```python
from build123d import *

# Parameters (mm, degrees)
BOSS_EXTRUDE2_DEPTH      = 10
SKETCH2_R                = 3
CUT_EXTRUDE1_DEPTH       = 5
CUT_EXTRUDE2_REACH       = 40.514
SKETCH3_R                = 1.5
SKETCH4_W                = 28.86751346
SKETCH4_H                = 120
SKETCH4_R                = 1.5
BOSS_EXTRUDE4_DEPTH      = 10
SKETCH5_R                = 3
CUT_EXTRUDE3_DEPTH       = 5
SKETCH6_W                = 4
SKETCH6_H                = 2
SKETCH6_W_2              = 2
SKETCH6_H_2              = 4
CUT_EXTRUDE4_DEPTH       = 4
SKETCH7_R                = 14.43375673
BOSS_EXTRUDE5_DEPTH      = 60
SKETCH8_R                = 9.43375673
CUT_EXTRUDE6_DEPTH       = 120
BOSS_EXTRUDE6_REACH      = 167.526
BOSS_EXTRUDE6_END_RADIUS = 14.43375673
SKETCH11_W               = 28.86751346
SKETCH11_H               = 10
CUT_EXTRUDE7_REACH       = 167.526
SKETCH13_W               = 18.86751346
SKETCH13_H               = 50
FILLET3_R                = 2
FILLET4_R                = 2


with BuildPart() as part:
    # Sketch1 → Boss-Extrude2 (new body)
    with BuildSketch(Plane.XY):
        Polygon((14.43375673, 25), (-14.43375673, 25), (-28.867513459, 0), (-14.43375673, -25), (14.43375673, -25), (28.867513459, 0), align=None)
    extrude(amount=BOSS_EXTRUDE2_DEPTH)

    # Sketch2 → Cut-Extrude1 (cut)
    with BuildSketch(Plane.XY.offset(10)):
        with Locations((-5.480077554, 5.480077554)):
            Circle(SKETCH2_R)
        with Locations((6.717514421, 6.717514421)):
            Circle(SKETCH2_R)
        with Locations((5.480077554, -5.480077554)):
            Circle(SKETCH2_R)
        with Locations((-6.717514421, -6.717514421)):
            Circle(SKETCH2_R)
    extrude(amount=-CUT_EXTRUDE1_DEPTH, mode=Mode.SUBTRACT)

    # Sketch3 → Cut-Extrude2 (cut, up to next)
    with BuildSketch(Plane.XY.offset(5), mode=Mode.PRIVATE) as cut_extrude2_sk1:
        with Locations((-5.480077554, 5.480077554)):
            Circle(SKETCH3_R)
    cut_extrude2_tool1 = extrude(cut_extrude2_sk1.sketch, amount=-CUT_EXTRUDE2_REACH, mode=Mode.PRIVATE) & part.part
    # Sketch3 → Cut-Extrude2 (cut, up to next)
    with BuildSketch(Plane.XY.offset(5), mode=Mode.PRIVATE) as cut_extrude2_sk2:
        with Locations((6.717514421, 6.717514421)):
            Circle(SKETCH3_R)
    cut_extrude2_tool2 = extrude(cut_extrude2_sk2.sketch, amount=-CUT_EXTRUDE2_REACH, mode=Mode.PRIVATE) & part.part
    # Sketch3 → Cut-Extrude2 (cut, up to next)
    with BuildSketch(Plane.XY.offset(5), mode=Mode.PRIVATE) as cut_extrude2_sk3:
        with Locations((5.480077554, -5.480077554)):
            Circle(SKETCH3_R)
    cut_extrude2_tool3 = extrude(cut_extrude2_sk3.sketch, amount=-CUT_EXTRUDE2_REACH, mode=Mode.PRIVATE) & part.part
    # Sketch3 → Cut-Extrude2 (cut, up to next)
    with BuildSketch(Plane.XY.offset(5), mode=Mode.PRIVATE) as cut_extrude2_sk4:
        with Locations((-6.717514421, -6.717514421)):
            Circle(SKETCH3_R)
    cut_extrude2_tool4 = extrude(cut_extrude2_sk4.sketch, amount=-CUT_EXTRUDE2_REACH, mode=Mode.PRIVATE) & part.part
    add(cut_extrude2_tool1.solids().sort_by_distance((-5.480078, 5.480078, 5))[0], mode=Mode.SUBTRACT)
    add(cut_extrude2_tool2.solids().sort_by_distance((6.717514, 6.717514, 5))[0], mode=Mode.SUBTRACT)
    add(cut_extrude2_tool3.solids().sort_by_distance((5.480078, -5.480078, 5))[0], mode=Mode.SUBTRACT)
    add(cut_extrude2_tool4.solids().sort_by_distance((-6.717514, -6.717514, 5))[0], mode=Mode.SUBTRACT)

    # Sketch4 → Boss-Extrude4 (add)
    with BuildSketch(Plane(origin=(0, 0, 0), x_dir=(-1, 0, 0), z_dir=(0, 0, -1))):
        with Locations((0, 85)):
            Rectangle(SKETCH4_W, SKETCH4_H)
        with Locations((0, 137)):
            Circle(SKETCH4_R, mode=Mode.SUBTRACT)
        with Locations((0, -85)):
            Rectangle(SKETCH4_W, SKETCH4_H)
        with Locations(Location((0, -137, 0), (0, 0, 180))):
            Circle(SKETCH4_R, mode=Mode.SUBTRACT)
    extrude(amount=-BOSS_EXTRUDE4_DEPTH)

    # Sketch5 → Cut-Extrude3 (cut)
    with BuildSketch(Plane.XY.offset(10)):
        with Locations((0, 137)):
            Circle(SKETCH5_R)
        with Locations((0, -137)):
            Circle(SKETCH5_R)
    extrude(amount=-CUT_EXTRUDE3_DEPTH, mode=Mode.SUBTRACT)

    # Sketch6 → Cut-Extrude4 (cut)
    with BuildSketch(Plane(origin=(0, 0, 0), x_dir=(-1, 0, 0), z_dir=(0, 0, -1))):
        with Locations((5, 137)):
            Rectangle(SKETCH6_W, SKETCH6_H)
        with Locations((0, 142)):
            Rectangle(SKETCH6_W_2, SKETCH6_H_2)
        with Locations((0, 132)):
            Rectangle(SKETCH6_W_2, SKETCH6_H_2)
        with Locations((-5, 137)):
            Rectangle(SKETCH6_W, SKETCH6_H)
        with Locations((0, -132)):
            Rectangle(SKETCH6_W_2, SKETCH6_H_2)
        with Locations((5, -137)):
            Rectangle(SKETCH6_W, SKETCH6_H)
        with Locations((-5, -137)):
            Rectangle(SKETCH6_W, SKETCH6_H)
        with Locations((0, -142)):
            Rectangle(SKETCH6_W_2, SKETCH6_H_2)
    extrude(amount=-CUT_EXTRUDE4_DEPTH, mode=Mode.SUBTRACT)



with BuildPart() as body_2:
    # Sketch7 → Boss-Extrude5 (new, symmetric)
    with BuildSketch(Plane(origin=(0, 0, 0), x_dir=(1, 0, 0), z_dir=(0, 1, 0))):
        with Locations(Location((0, -70, 0), (0, 0, 270))):
            Circle(SKETCH7_R)
    extrude(amount=BOSS_EXTRUDE5_DEPTH, both=True)

    # Sketch8 → Cut-Extrude6 (cut)
    with BuildSketch(Plane.XZ.offset(60)):
        with Locations(Location((0, 70, 0), (0, 0, 270))):
            Circle(SKETCH8_R)
    extrude(amount=-CUT_EXTRUDE6_DEPTH, mode=Mode.SUBTRACT)


with BuildPart() as part_1:
    add(part.part)

    add(body_2.part)  # Boss-Extrude6 merges body 2
    # Boss-Extrude6: up to this cylinder (the profile starts outside it)
    boss_extrude6_end = Plane(origin=(0, 55, 70), z_dir=(0, -1, 0)) * Cylinder(BOSS_EXTRUDE6_END_RADIUS, 364.919513459, mode=Mode.PRIVATE)
    # Sketch11 → Boss-Extrude6 (add, up to the surface)
    with BuildSketch(Plane.XY.offset(10), mode=Mode.PRIVATE) as boss_extrude6_sk1:
        with Locations((0, 55)):
            Rectangle(SKETCH11_W, SKETCH11_H)
    boss_extrude6_tool1 = extrude(boss_extrude6_sk1.sketch, amount=BOSS_EXTRUDE6_REACH, mode=Mode.PRIVATE) - boss_extrude6_end
    boss_extrude6 = boss_extrude6_tool1.solids().sort_by_distance((0, 55, 10))[0]
    add(boss_extrude6)

    # Mirror1: Boss-Extrude6 across plane
    add(boss_extrude6.mirror(Plane.ZX))

    # Sketch13 → Cut-Extrude7 (cut, up to next)
    with BuildSketch(Plane.XY.offset(10), mode=Mode.PRIVATE) as cut_extrude7_sk1:
        with Locations((0, 102.5)):
            Rectangle(SKETCH13_W, SKETCH13_H)
    cut_extrude7_tool1 = extrude(cut_extrude7_sk1.sketch, amount=-CUT_EXTRUDE7_REACH, mode=Mode.PRIVATE) & part_1.part
    # Sketch13 → Cut-Extrude7 (cut, up to next)
    with BuildSketch(Plane.XY.offset(10), mode=Mode.PRIVATE) as cut_extrude7_sk2:
        with Locations((0, -102.5)):
            Rectangle(SKETCH13_W, SKETCH13_H)
    cut_extrude7_tool2 = extrude(cut_extrude7_sk2.sketch, amount=-CUT_EXTRUDE7_REACH, mode=Mode.PRIVATE) & part_1.part
    add(cut_extrude7_tool1.solids().sort_by_distance((0, 102.5, 10))[0], mode=Mode.SUBTRACT)
    add(cut_extrude7_tool2.solids().sort_by_distance((0, -102.5, 10))[0], mode=Mode.SUBTRACT)

    # Fillet3
    fillet3_edges = [part_1.edges().sort_by_distance(p)[0] for p in [
        (28.867513459, 0, 5),
        (14.43375673, -25, 5),
        (-14.43375673, -25, 5),
        (-28.867513459, 0, 5),
        (-14.43375673, 25, 5),
        (14.43375673, 25, 5),
        (14.43375673, 60, 40),
        (-14.43375673, 60, 40),
        (10.206207262, 60, 80.206207262),
        (10.206207262, -60, 80.206207262),
        (-14.43375673, -60, 40),
        (14.43375673, -60, 40),
        (-9.43375673, 77.5, 5),
        (-9.43375673, 127.5, 5),
        (9.43375673, 127.5, 5),
        (9.43375673, 77.5, 5),
        (9.43375673, -77.5, 5),
        (9.43375673, -127.5, 5),
        (-9.43375673, -127.5, 5),
        (-9.43375673, -77.5, 5),
        (14.43375673, 145, 5),
        (-14.43375673, 145, 5),
        (14.43375673, -145, 5),
        (-14.43375673, -145, 5),
    ]]
    fillet(fillet3_edges, radius=FILLET3_R)

    # Fillet4
    fillet4_edges = [part_1.edges().sort_by_distance(p)[0] for p in [
        (14.43375673, 37.767949192, 10),
        (-14.43375673, 100.5, 10),
        (-14.43375673, -37.767949192, 10),
        (14.43375673, -100.5, 10),
        (-14.43375673, 37.767949192, 10),
        (14.43375673, 100.5, 10),
        (21.495934556, 12.767949192, 10),
        (0, 145, 10),
        (-21.495934556, 12.767949192, 10),
        (-21.495934556, -12.767949192, 10),
        (14.43375673, -37.767949192, 10),
        (21.495934556, -12.767949192, 10),
        (-14.43375673, -100.5, 10),
        (0, -145, 10),
        (14.501905077, 25.018260295, 10),
        (-14.501905077, 25.018260295, 10),
        (-14.501905077, -25.018260295, 10),
        (14.501905077, -25.018260295, 10),
        (13.847970292, 144.414213562, 10),
        (-13.847970292, 144.414213562, 10),
        (28.558112383, 0, 10),
        (-28.558112383, 0, 10),
        (13.847970292, -144.414213562, 10),
        (-13.847970292, -144.414213562, 10),
    ]]
    fillet(fillet4_edges, radius=FILLET4_R)


solid = part_1.part
```
Part model, mm, in its own coordinate system. A direction names the side the tool comes from. Give positions to 0.01 mm unless a question says otherwise; leave off trailing zeros. Loops run counter-clockwise (first coordinate to the right, second up) from the corner with the lowest first, then second, coordinate; pieces in that order, holes last. Notation, with made-up numbers: M 16,-6.5 L 66,-6.5 A6 cw 66,0.5 Z; hole C 72,-5 d2. An arc over 180 degrees is marked long. Return JSON: item names as keys, results as strings.
1) Pull direction Z, two halves, no side cores. Call faces 6 (the face through (-21.591, -12.603, 3.944)), 7 (the face through (11, -101, 10)), 8 (the face through (0, 50, 32)): released by +Z, released by -Z, zero draft, split by the parting line, or undercut.
Calculated:
{"face 6": "zero draft", "face 7": "released by +Z", "face 8": "undercut"}
2) Flat gauge pins, fed straight in: pin 1 Ø3 at (y, z) = (58.5, 56) entering from +X; pin 2 Ø2 at (x, y) = (-0.5, 133) entering from -Z; pin 3 Ø8 at (y, z) = (93.5, 5.5) entering from -X; pin 4 Ø3 at (x, y) = (-7.5, -5.5) entering from +Z. Where does each tip first touch, or does it go through?
Calculated:
{"pin 1": "stops at x = 14.43", "pin 2": "stops at z = 0", "pin 3": "stops at x = -14.43", "pin 4": "stops at z = 83.13"}
3) Saw through at D-D, the plane z = 67. List the corners of the cut face in (x, y).
Calculated:
{"outline": "M -14.43,-58 A2 ccw -12.43,-60 L -8.94,-60 L -8.94,60 L -12.43,60 A2 ccw -14.43,58 L -14.43,50 L -14.12,50 L -14.12,-50 L -14.43,-50 Z; M 8.94,-60 L 12.43,-60 A2 ccw 14.43,-58 L 14.43,-50 L 14.12,-50 L 14.12,50 L 14.43,50 L 14.43,58 A2 ccw 12.43,60 L 8.94,60 Z"}
4) 3-axis set-ups, long thin cutter, end or side, ignore diameter. For faces 1 (the face through (1.61, -134.47, 7.54)), 2 (the face through (5, 6, 5)), 3 (the face through (-9.434, 102, 5)), 4 (the face through (0, -60, 38)), 5 (the face through (14.434, 75, 6)): which of +Z, -Z, +X, -X, +Y, -Y reach the whole face in a straight line?
Calculated:
{"face 1": "+Z", "face 2": "none", "face 3": "+Z, -Z", "face 4": "+Z, +X, -X, -Y", "face 5": "+Z, -Z, +X, +Y"}
5) Drill centre lines: line 1 (Y direction, x = -10, z = 47); line 2 (X direction, y = 52, z = 70.5); line 3 (Z direction, x = -1.5, y = -27.5). Where is each one in solid material? Low to high.
Calculated:
{"line 1": "y = -60 to -50, 50 to 60", "line 2": "x = -14.43 to -9.42, 9.42 to 14.43", "line 3": "z = 0 to 10, 55.64 to 60.69, 79.31 to 84.36"}
6) Saw through at C-C, the plane y = 88. List the corners of the cut face in (x, z).
Calculated:
{"outline": "M -14.43,0 L -9.43,0 L -9.43,10 L -12.43,10 A2 ccw -14.43,8 Z; M 9.43,0 L 14.43,0 L 14.43,8 A2 ccw 12.43,10 L 9.43,10 Z"}
7) Saw through at A-A, the plane z = 25.5. List the corners of the cut face in (x, y), then the cut area to 3 significant figures.
Calculated:
{"outline": "M -14.43,-58 A2 ccw -12.43,-60 L 12.43,-60 A2 ccw 14.43,-58 L 14.43,-50 L -14.43,-50 Z; M -14.43,50 L 14.43,50 L 14.43,58 A2 ccw 12.43,60 L -12.43,60 A2 ccw -14.43,58 Z", "area": "574 mm2"}
8) Saw through at B-B, the plane y = -44. List the corners of the cut face in (x, z), then the cut area to 3 significant figures.
Calculated:
{"outline": "M -14.43,0 L 14.43,0 L 14.43,8 A2 ccw 12.43,10 L -12.43,10 A2 ccw -14.43,8 Z; C 0,70 d28.87; hole C 0,70 d18.87", "area": "662 mm2"}
